Design review of the part built by this model. Coordinates are the model's own, in mm. Face numbers are marked on the shaded views. A direction names the side the tool comes from. Round coordinates to 2 decimals unless told otherwise and drop trailing zeros. Loops run counter-clockwise (first coordinate to the right, second up) from the corner with the lowest first, then second, coordinate; pieces in that order, holes last. Notation, with made-up numbers: M -14.5,42.25 L 29.5,42.25 A20 cw 29.5,79.25 Z; hole C 4.25,34 d1. An arc over 180 degrees is marked long. Use a Markdown table: item, result.
from build123d import *

# Parameters (mm, degrees)
SKETCH_W           = 60
SKETCH_H           = 60
PAD_DEPTH          = 5
COPYSKETCH001_W    = 50
COPYSKETCH001_H    = 50
POCKET_DEPTH       = 11
COPYSKETCH002001_W = 20
COPYSKETCH002001_H = 18
PAD001_DEPTH       = 25


with BuildPart() as part:
    # Sketch → Pad (new body)
    with BuildSketch(Plane.XY):
        with Locations((22.847713, -14.499916)):
            Rectangle(SKETCH_W, SKETCH_H)
    extrude(amount=PAD_DEPTH)

    # CopySketch001 → Pocket (cut)
    with BuildSketch(Plane(origin=(0, 0, 0), x_dir=(1, 0, 0), z_dir=(0, 0, -1))):
        with Locations((22.847713, 14.499916)):
            Rectangle(COPYSKETCH001_W, COPYSKETCH001_H)
    extrude(amount=-POCKET_DEPTH, mode=Mode.SUBTRACT)

    # CopySketch002001 → Pad001 (join)
    with BuildSketch(Plane(origin=(0, 0, 0), x_dir=(1, 0, 0), z_dir=(0, 0, -1))):
        with Locations((7.847713, 30.499916)):
            Rectangle(COPYSKETCH002001_W, COPYSKETCH002001_H)
        with Locations((37.847713, 30.499916)):
            Rectangle(COPYSKETCH002001_W, COPYSKETCH002001_H)
        with Locations((37.847713, -1.500084)):
            Rectangle(COPYSKETCH002001_W, COPYSKETCH002001_H)
        with Locations((7.847713, -1.500084)):
            Rectangle(COPYSKETCH002001_W, COPYSKETCH002001_H)
    extrude(amount=-PAD001_DEPTH)


solid = part.part
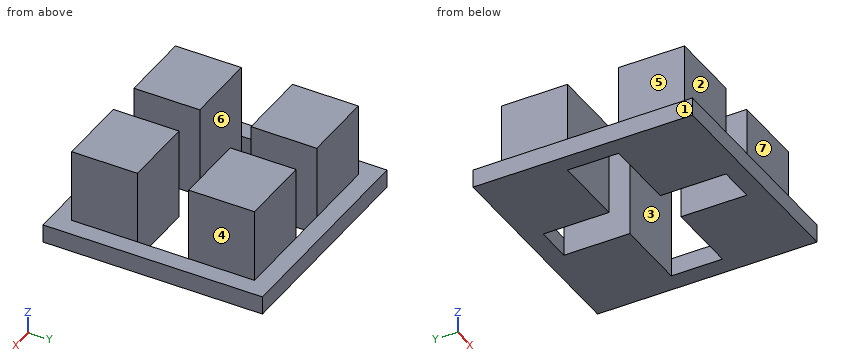
1. Take a section at A-A on y = -14. Give the boundary of the cut face in (x, z).
Check values:
| item | result |
|---|---|
| outline | M -7.15,0 L -2.15,0 L -2.15,5 L -7.15,5 Z; M 47.85,0 L 52.85,0 L 52.85,5 L 47.85,5 Z |
2. Machinability: for the marked faces 4, 5, 6 and 7, which of the approach directions +Z, -Z, +X, -X, +Y, -Y give a long, thin tool a straight path to every point of the face, cutting with its end or side? Answer none if there is none.
Check values:
| item | result |
|---|---|
| face 4 | +Z, +X, +Y, -Y |
| face 5 | +Z, -X, +Y, -Y |
| face 6 | +Z, -Z |
| face 7 | +Z, +X, -X, -Y |
3. The part is to be moulded in two halves that separate along Y. For the marked faces 1, 2 and 3, say which applies: pulls with the +Y half, pulls with the -Y half, needs draft (parallel to the pull), parting line crosses it, or undercut.
Check values:
| item | result |
|---|---|
| face 1 | needs draft |
| face 2 | pulls with the -Y half |
| face 3 | undercut |
4. Take a section at B-B on z = 7.25. Give the boundary of the cut face in (x, y).
Check values:
| item | result |
|---|---|
| outline | M -2.15,-39.5 L 17.85,-39.5 L 17.85,-21.5 L -2.15,-21.5 Z; M -2.15,-7.5 L 17.85,-7.5 L 17.85,10.5 L -2.15,10.5 Z; M 27.85,-39.5 L 47.85,-39.5 L 47.85,-21.5 L 27.85,-21.5 Z; M 27.85,-7.5 L 47.85,-7.5 L 47.85,10.5 L 27.85,10.5 Z |
5. Take a section at C-C on x = 9.5. Give the boundary of the cut face in (y, z), and give its area (3 significant figures).
Check values:
| item | result |
|---|---|
| outline | M -44.5,0 L -21.5,0 L -21.5,25 L -39.5,25 L -39.5,5 L -44.5,5 Z; M -7.5,0 L 15.5,0 L 15.5,5 L 10.5,5 L 10.5,25 L -7.5,25 Z |
| area | 950 mm² |
6. Take a section at D-D on y = -23. Give the boundary of the cut face in (x, z).
Check values:
| item | result |
|---|---|
| outline | M -7.15,0 L 17.85,0 L 17.85,25 L -2.15,25 L -2.15,5 L -7.15,5 Z; M 27.85,0 L 52.85,0 L 52.85,5 L 47.85,5 L 47.85,25 L 27.85,25 Z |
7. Insertion check: pin 1 (10 mm diameter, centred on y = -35.5, z = 21, fed in from +X); pin 2 (5.5 mm diameter, centred on y = 4.5, z = 17.5, fed in from -X); pin 3 (6 mm diameter, centred on x = 3.5, z = 15, fed in from -Y). Each pin has a flat end and moves straight along its axis. Give the tip position at first contact, or say it passes through.
Check values:
| item | result |
|---|---|
| pin 1 | stops at x = 47.85 |
| pin 2 | stops at x = -2.15 |
| pin 3 | stops at y = -39.5 |
8. Wall thickness on line 1 along Y through (x, z) = (43.5, 1.75); line 2 along X through (y, z) = (4, 14.25); line 3 along Y through (x, z) = (25, 2.5): over which ranges is each line inside the solid? List them lowest first. Write a range as from..to.
Check values:
| item | result |
|---|---|
| line 1 | y = -44.5..-21.5, -7.5..15.5 |
| line 2 | x = -2.15..17.85, 27.85..47.85 |
| line 3 | y = -44.5..-39.5, 10.5..15.5 |
